from build123d import *

# Parameters (mm, degrees)
SKETCH2_R   = 16
SKETCH2_R_2 = 12


with BuildPart() as part:
    # Sweep1: sweep along a path in Sketch1
    with BuildLine(Plane(origin=(0, 0, 0), x_dir=(1, 0, 0), z_dir=(0, 1, 0))) as sweep1_path:
        Line((0, 0), (-70.1970105, 0))
        ThreePointArc((-70.1970105, 0), (-98.652281007, 8.886771224), (-116.99253235, 32.388096786))
        Line((-116.99253235, 32.388096786), (-132.496272122, 73.582145179))
        ThreePointArc((-132.496272122, 73.582145179), (-129.748156844, 132.804715841), (-84.855924311, 171.528771306))
        Line((-84.855924311, 171.528771306), (10.197010652, 201.498846579))
    # Sketch2 → Sweep1 (sweep)
    with BuildSketch(Plane(origin=(0, 0, 0), x_dir=(0, 0, -1), z_dir=(1, 0, 0))):
        Circle(SKETCH2_R)
        Circle(SKETCH2_R_2, mode=Mode.SUBTRACT)
    sweep(path=sweep1_path.line)


solid = part.part
Part model, mm, in its own coordinate system. A direction names the side the tool comes from. Give positions to 0.01 mm unless a question says otherwise; leave off trailing zeros. Loops run counter-clockwise (first coordinate to the right, second up) from the corner with the lowest first, then second, coordinate; pieces in that order, holes last.
(1) Band-saw the part on B-B (x = -58). Count the separate pieces of the cut face and the enclosed holes in it, and give its area (3 significant figures).
Return value:
separate pieces: 2
enclosed holes: 2
area: 721 mm2
(2) Band-saw the part on A-A (y = 0). Write the cut outline in (x, z), and give its area (3 significant figures).
Return value:
outline: (-147.47, -67.95) arc R91 ccw to (-89.67, -186.79) - (5.39, -216.76) - (6.59, -212.94) - (-88.46, -182.97) arc R87 cw to (-143.73, -69.36) - (-128.22, -28.16) arc R62 cw to (-70.2, 12) - (0, 12) - (0, 16) - (-70.2, 16) arc R66 ccw to (-131.97, -26.75) - close; (-121.27, -77.81) arc R63 ccw to (-81.25, -160.08) - (13.81, -190.05) - (15.01, -186.24) - (-80.04, -156.27) arc R59 cw to (-117.52, -79.22) - (-102.02, -38.02) arc R34 cw to (-70.2, -16) - (0, -16) - (0, -12) - (-70.2, -12) arc R38 ccw to (-105.76, -36.61) - close
area: 3,170 mm2
(3) Pull direction Z, two halves, no side cores. Call faces 1 (the flat face through (8.438, -10.741, -207.079)), 2 (the cylindrical face through (-133.765, 7.302, -49.919)), 3 (the flat face through (0, -12, 2)): pulls with the +Z half, pulls with the -Z half, needs draft (parallel to the pull), parting line crosses it, or undercut.
Return value:
face 1: pulls with the -Z half
face 2: undercut
face 3: needs draft
(4) Pin check, flat tips, straight feed: pin 1 (6 mm diameter, centred on y = -0.5, z = -131.5, fed in from +X); pin 2 (3 mm diameter, centred on x = -118.5, y = 0.5, fed in from +Z); pin 3 (8 mm diameter, centred on x = -28, y = 1.5, fed in from -Z). Stop position of each tip, or through.
Return value:
pin 1: stops at x = -110.17
pin 2: stops at z = -3.48
pin 3: stops at z = -207.45
(5) 3-axis set-ups, long thin cutter, end or side, ignore diameter. For faces 4 (the cylindrical face through (-35.59, 15.62, 3.47)), 5 (the cylindrical face through (-111.02, 6.13, -58.48)): which of +Z, -Z, +X, -X, +Y, -Y reach the whole face in a straight line?
Return value:
face 4: +X
face 5: none
(6) Drill centre lines: line 1 along Y through (x, z) = (-15.5, 0); line 2 along Z through (x, y) = (-60, 8); line 3 along Z through (x, y) = (-46, -6.5). Where is each one in solid material? Low to high.
Return value:
line 1: y = -16 to -12, 12 to 16
line 2: z = -193.89 to -188.74, -169.99 to -164.84, -13.86 to -8.94, 8.94 to 13.86
line 3: z = -199.11 to -194.36, -173.2 to -168.45, -14.62 to -10.09, 10.09 to 14.62
